The model under review builds one solid part; all positions refer to its coordinate system, in mm. A direction names the side the tool comes from. Coordinates: 2 decimals unless noted, no trailing zeros. Order: outer loops, then holes, each group sorted by start corner. A loop starts at its lowest first (then second) coordinate and runs counter-clockwise, first axis right, second up.
```python
from build123d import *

# Parameters (mm, degrees)
F0_W     = 4.5
F0_H     = 40
F0_W_2   = 45
F0_H_2   = 10
F1_DEPTH = 1.5
F2_R     = 2.5
F3_DEPTH = 25
F4_W     = 33
F4_H     = 58
F5_DEPTH = 17


with BuildPart() as f1:
    # F0 (on Top) → F1 (new body)
    with BuildSketch(Plane.XY):
        with Locations((24.75, 0)):
            Rectangle(F0_W, F0_H)
        Rectangle(F0_W_2, F0_H)
        with Locations((0, 25)):
            Rectangle(F0_W_2, F0_H_2)
        with Locations((-24.75, 0)):
            Rectangle(F0_W, F0_H)
        with Locations((0, -25)):
            Rectangle(F0_W_2, F0_H_2)
    extrude(amount=F1_DEPTH)

    # F2 (on face) → F3 (cut)
    with BuildSketch(Plane.XY.offset(1.5)):
        with Locations((-21.5, 14.5)):
            Circle(F2_R)
        with Locations((21.5, 14.5)):
            Circle(F2_R)
        with Locations((21.5, -14.5)):
            Circle(F2_R)
        with Locations((-21.5, -14.5)):
            Circle(F2_R)
    extrude(amount=-F3_DEPTH, mode=Mode.SUBTRACT)

    # F4 (on face) → F5 (join)
    with BuildSketch(Plane.XY.offset(1.5)):
        Rectangle(F4_W, F4_H)
    extrude(amount=F5_DEPTH)


solid = f1.part
```
(1) Machinability: for faces 4 (the face through (16.5, 0, 10)), 5 (the face through (0, -29, 10)), 6 (the face through (25, 20, 1)), 7 (the face through (-25, 20, 1)), which of the approach directions +Z, -Z, +X, -X, +Y, -Y give a long, thin tool a straight path to every point of the face, cutting with its end or side? Answer none if there is none.
A:
face 4: +Z, +X, +Y, -Y
face 5: +Z, +X, -X, -Y
face 6: +Z, -Z, +X, +Y
face 7: +Z, -Z, -X, +Y
(2) We need section B-B, the plane x = 21.5. Write out the cut boundary in (y, z).
A:
outline: (-30, 0) - (-17, 0) - (-17, 1.5) - (-30, 1.5) - close; (-12, 0) - (12, 0) - (12, 1.5) - (-12, 1.5) - close; (17, 0) - (30, 0) - (30, 1.5) - (17, 1.5) - close
(3) We need section D-D, the plane x = 5.5. Write out the cut boundary in (y, z), and give its area (3 significant figures).
A:
outline: (-30, 0) - (30, 0) - (30, 1.5) - (29, 1.5) - (29, 18.5) - (-29, 18.5) - (-29, 1.5) - (-30, 1.5) - close
area: 1,080 mm2
(4) We need section A-A, the plane y = -14.5. Write out the cut boundary in (x, z), and give its area (3 significant figures).
A:
outline: (-27, 0) - (-24, 0) - (-24, 1.5) - (-27, 1.5) - close; (-19, 0) - (19, 0) - (19, 1.5) - (16.5, 1.5) - (16.5, 18.5) - (-16.5, 18.5) - (-16.5, 1.5) - (-19, 1.5) - close; (24, 0) - (27, 0) - (27, 1.5) - (24, 1.5) - close
area: 627 mm2
(5) Draft analysis for pull direction Y (two halves, no side actions). For faces 1 (the face through (-25, -20, 1)), 2 (the face through (-24, 14.6, 0.8)), 3 (the face through (22.5, 25, 1)), state which applies: released by +Y, released by -Y, zero draft, split by the parting line, or undercut.
A:
face 1: released by -Y
face 2: undercut
face 3: zero draft
(6) For pin 1 Ø1.6 at (x, z) = (-24, 1) entering from -Y; pin 2 Ø8.5 at (y, z) = (3.5, 9.5) entering from +X; pin 3 Ø1.6 at (y, z) = (-23, 0.5) entering from +X; pin 4 Ø4.5 at (x, y) = (21.5, -14.5) entering from -Z, all flat-tipped, find the tip position at first contact; note any pin that passes through.
A:
pin 1: stops at y = -20
pin 2: stops at x = 16.5
pin 3: stops at x = 22.5
pin 4: passes through
(7) Wall thickness on probe 1 along Y at (x, z) = (-21.5, 0.65); probe 2 along Z at (x, y) = (-20, 20); probe 3 along Y at (x, z) = (-7.5, 2.5): over which ranges is each line inside the solid? List them lowest first.
A:
probe 1: y = -30 to -17, -12 to 12, 17 to 30
probe 2: z = 0 to 1.5
probe 3: y = -29 to 29
(8) We need section C-C, the plane y = 0.5. Write out the cut boundary in (x, z).
A:
outline: (-27, 0) - (27, 0) - (27, 1.5) - (16.5, 1.5) - (16.5, 18.5) - (-16.5, 18.5) - (-16.5, 1.5) - (-27, 1.5) - close
